from build123d import *

# Parameters (mm, degrees)
ESQUISSE1_W                  = 32
ESQUISSE1_H                  = 32
BOSS_EXTRU_1_DEPTH           = 20
ENL_V_MAT_EXTRU_1_DEPTH      = 50.477267507
ENL_V_MAT_EXTRU_1_DEPTH_BACK = 50.477267507
ESQUISSE2_R                  = 12.8
BOSS_EXTRU_2_DEPTH           = 20
ESQUISSE4_R                  = 3.25
ENL_V_MAT_EXTRU_2_DEPTH      = 10
ENL_V_MAT_EXTRU_3_DEPTH      = 20
ESQUISSE6_W                  = 20
ESQUISSE6_H                  = 20
ESQUISSE6_R                  = 8.1
BOSS_EXTRU_3_DEPTH           = 20
CHANFREIN1_SIZE              = 6
CHANFREIN2_SIZE              = 2
ENL_V_START                  = -2
ESQUISSE7_R                  = 8.1
ENL_V_MAT_EXTRU_4_DEPTH      = 2


with BuildPart() as part:
    # Esquisse1 → Boss.-Extru.1 (new body)
    with BuildSketch(Plane.XY):
        with Locations((16, 16)):
            Rectangle(ESQUISSE1_W, ESQUISSE1_H)
    extrude(amount=BOSS_EXTRU_1_DEPTH)

    # Esquisse2 → Enlèv. mat.-Extru.1 (cut, two sides: drawn at the far end of the back side and taken through both)
    with BuildSketch(Plane.XY.offset(20).offset(-ENL_V_MAT_EXTRU_1_DEPTH_BACK)):
        with Locations((16, 16)):
            Circle(ESQUISSE2_R)
    extrude(amount=ENL_V_MAT_EXTRU_1_DEPTH + ENL_V_MAT_EXTRU_1_DEPTH_BACK, mode=Mode.SUBTRACT)

    # Esquisse3 → Boss.-Extru.2 (add)
    with BuildSketch(Plane.XY.offset(20)):
        Polygon((0, 0), (0, 32), (-13, 23), (-13, 9), align=None)
    extrude(amount=-BOSS_EXTRU_2_DEPTH)

    # Esquisse4 → Enlèv. mat.-Extru.2 (cut)
    with BuildSketch(Plane.ZY.offset(13)):
        with Locations((10, 16)):
            Circle(ESQUISSE4_R)
    extrude(amount=-ENL_V_MAT_EXTRU_2_DEPTH, mode=Mode.SUBTRACT)

    # Esquisse5 → Enlèv. mat.-Extru.3 (cut)
    with BuildSketch(Plane.ZY.offset(3)):
        Polygon((12.973353886, 10.85), (15.946707773, 16), (12.973353886, 21.15), (7.026646114, 21.15), (4.053292227, 16), (7.026646114, 10.85), align=None)
    extrude(amount=-ENL_V_MAT_EXTRU_3_DEPTH, mode=Mode.SUBTRACT)

    # Esquisse6 → Boss.-Extru.3 (add)
    with BuildSketch(Plane(origin=(32, 0, 0), x_dir=(0, 0, -1), z_dir=(1, 0, 0))):
        with Locations((-10, 16)):
            Rectangle(ESQUISSE6_W, ESQUISSE6_H)
        with Locations((-10, 16)):
            Circle(ESQUISSE6_R, mode=Mode.SUBTRACT)
    extrude(amount=BOSS_EXTRU_3_DEPTH)

    # Chanfrein1
    chanfrein1_edges = [part.edges().sort_by_distance(p)[0] for p in [
        (32, 6, 10),
        (32, 26, 10),
    ]]
    chamfer(chanfrein1_edges, length=CHANFREIN1_SIZE - 0.0001)  # a hair under: the kernel refuses the full size

    # Chanfrein2
    chanfrein2_edges = [part.edges().sort_by_distance(p)[0] for p in [
        (44.99995, 6, 20),
        (44.99995, 6, 0),
        (44.99995, 26, 0),
        (44.99995, 26, 20),
    ]]
    chamfer(chanfrein2_edges, length=CHANFREIN2_SIZE)

    # Esquisse7 → Enlèv. mat.-Extru.4 (cut)
    with BuildSketch(Plane(origin=(32, 0, 0), x_dir=(0, 0, -1), z_dir=(1, 0, 0)).offset(ENL_V_START)):
        with Locations((-10, 16)):
            Circle(ESQUISSE7_R)
    extrude(amount=ENL_V_MAT_EXTRU_4_DEPTH, mode=Mode.SUBTRACT)


solid = part.part
Can you work these out from the model? Positions are in its coordinate system, mm. A direction names the side the tool comes from. Give positions to 0.01 mm unless a question says otherwise; leave off trailing zeros. Loops run counter-clockwise (first coordinate to the right, second up) from the corner with the lowest first, then second, coordinate; pieces in that order, holes last. Notation, with made-up numbers: M -25.75,-28.75 L 28.25,-28.75 A26 cw 28.25,-4.75 Z; hole C -13.5,78.5 d4. An arc over 180 degrees is marked long. One line per item, written item: value. Start each with the question number.
1) Thinking about a two-plate mould opening in X: for faces 1 (the face through (45, 26, 10)), 2 (the face through (1, 21.15, 10)), 3 (the face through (0.59, 18.54, 14.48)), 4 (the face through (-6.41, 27.56, 10.14)), which applies, +X half, -X half, draft (parallel to the pull), parting line (faces both ways), or undercut?
2) I'm going to push flat-ended pins straight in: pin 1 (2 mm diameter, centred on y = 18, z = 4.5, fed in from +X); pin 2 (4 mm diameter, centred on x = 42.5, z = 6, fed in from +Y); pin 3 (4 mm diameter, centred on y = 16, z = 10, fed in from -X). Where does each tip first touch, or does it pass through?
3) If we section it at B-B, the plane x = 44.5: Write out the boundary of the cut face in (y, z).
4) On a 3-axis mill with a long thin cutter (end or side, diameter ignored), from which of +Z, -Z, +X, -X, +Y, -Y can I reach the whole of each face in a straight line? I mean faces 5 (the face through (45, 7, 1)), 6 (the face through (16, 0, 10)), 7 (the face through (45, 6, 10)), 8 (the face through (-3, 14, 13)), 9 (the face through (-8.07, 18.197, 7.605)). Say none if no direction works.
5) If we section it at D-D, the plane y = 14: Write out the boundary of the cut face in (x, z).
6) If I drill on line 1 (Y direction, x = 39.75, z = 10); line 2 (X direction, y = 16, z = 5.5); line 3 (X direction, y = 16, z = 9.75), over which ranges is the centre line in solid material (lowest first)? Write a range as [from, to].
7) If we section it at A-A, the plane x = 16: Write out the boundary of the cut face in (y, z).
Completed:
1. face 1: draft
1. face 2: undercut
1. face 3: undercut
1. face 4: -X half
2. pin 1: stops at x = 30
2. pin 2: stops at y = 26
2. pin 3: stops at x = 28.64
3. outline: M 6,2 L 8,0 L 24,0 L 26,2 L 26,18 L 24,20 L 8,20 L 6,18 Z; hole C 16,10 d16.2
4. face 5: -Z, +X, -Y
4. face 6: +Z, -Z, +X, -X, -Y
4. face 7: +Z, -Z, +X, -Y
4. face 8: none
4. face 9: -X
5. outline: M -13,0 L 3.36,0 L 3.36,5.21 L -3,5.21 L -3,7.44 L -13,7.44 Z; M -13,12.56 L -3,12.56 L -3,14.79 L 3.36,14.79 L 3.36,20 L -13,20 Z; M 28.64,0 L 52,0 L 52,2.15 L 30,2.15 L 30,17.85 L 52,17.85 L 52,20 L 28.64,20 Z
6. line 1: y = [6, 7.9], [24.1, 26]
6. line 2: x = [-13, -3], [28.8, 30]
6. line 3: x = [28.8, 30]
7. outline: M 0,0 L 3.2,0 L 3.2,20 L 0,20 Z; M 28.8,0 L 32,0 L 32,20 L 28.8,20 Z
